Can you work these out from the drawing? Everything is in mm from the part's minimum corner. Give positions to 0.01 mm unless a question says otherwise; leave off trailing zeros. Write each loop counter-clockwise with the first axis right and the second up, starting at its lowest first coordinate (ties: lowest second). Pieces come first, ordered by that corner, then holes. Notation, with made-up numbers: (85, 45.25) - (131, 45.25) arc R22 cw to (131, 72.25) - close; hole circle Ø8 at (2, -1). An arc over 180 degrees is marked (long way). Use a Markdown table: item, result.
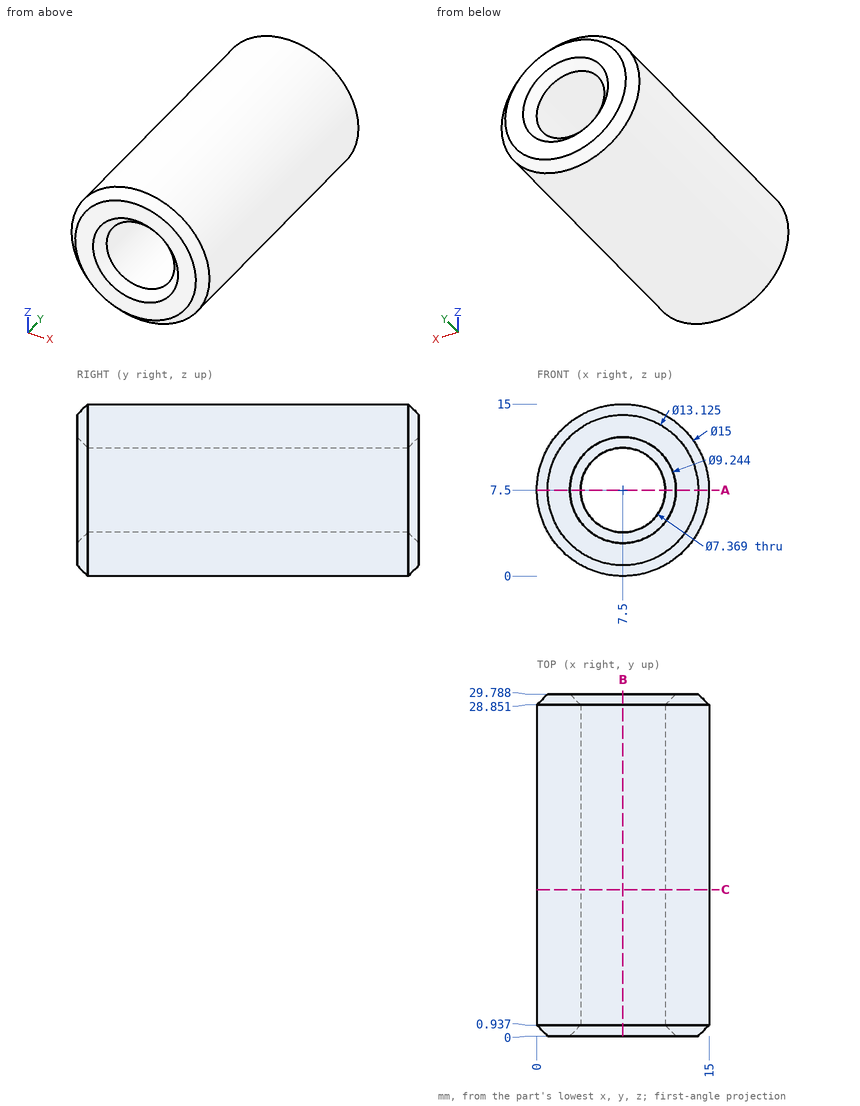
Item 1: If we section it at B-B, the plane x = 7.5: Write out the boundary of the cut face in (y, z) (1 decimal).
Values:
| item | result |
|---|---|
| outline | (0, 0.9) - (0.9, 0) - (28.9, 0) - (29.8, 0.9) - (29.8, 2.9) - (28.9, 3.8) - (0.9, 3.8) - (0, 2.9) - close; (0, 12.1) - (0.9, 11.2) - (28.9, 11.2) - (29.8, 12.1) - (29.8, 14.1) - (28.9, 15) - (0.9, 15) - (0, 14.1) - close |
Item 2: If we section it at A-A, the plane z = 7.5: Write out the boundary of the cut face in (x, y) (1 decimal).
Values:
| item | result |
|---|---|
| outline | (0, 0.9) - (0.9, 0) - (2.9, 0) - (3.8, 0.9) - (3.8, 28.9) - (2.9, 29.8) - (0.9, 29.8) - (0, 28.9) - close; (11.2, 0.9) - (12.1, 0) - (14.1, 0) - (15, 0.9) - (15, 28.9) - (14.1, 29.8) - (12.1, 29.8) - (11.2, 28.9) - close |
Item 3: Will these pins go through, and if not, where does the flat tip stop? pin 1 Ø2 at (x, y) = (5.5, 3) entering from -Z; pin 2 Ø2 at (x, y) = (5.5, 4.5) entering from +Z; pin 3 Ø1 at (x, y) = (3, 13.5) entering from -Z (1 decimal).
Values:
| item | result |
|---|---|
| pin 1 | stops at z = 0.07 |
| pin 2 | stops at z = 14.93 |
| pin 3 | stops at z = 1.2 |
Item 4: I need wall thicknesses on line 1 along X through (y, z) = (10.75, 7.5) (1 decimal); line 2 along X through (y, z) = (15.5, 6.75). Which ranges of each line are inside material? Lowest first, please. Write a range as [from, to].
Values:
| item | result |
|---|---|
| line 1 | x = [0, 3.8], [11.2, 15] |
| line 2 | x = [0.04, 3.89], [11.11, 14.96] |
Item 5: If we section it at C-C, the plane y = 12.75: Write out the boundary of the cut face in (x, z) (1 decimal), plus the area to 3 significant figures.
Values:
| item | result |
|---|---|
| outline | circle Ø15 at (7.5, 7.5); hole circle Ø7.4 at (7.5, 7.5) |
| area | 134 mm2 |
